```python
from build123d import *

# Parameters (mm, degrees)
SKETCH1_R           = 0.635
BOSS_EXTRUDE1_DEPTH = 1.27
FILLET1_R           = 0.254


with BuildPart() as part:
    # Sketch1 → Boss-Extrude1 (new body)
    with BuildSketch(Plane(origin=(0, 0, 0), x_dir=(1, 0, 0), z_dir=(0, 1, 0))):
        with BuildLine():
            ThreePointArc((-4.445, -13.249953655), (-4.662189736, -11.349360189), (-5.931882655, -9.9185189))
            ThreePointArc((-5.931882655, -9.9185189), (0, 11.557), (5.931882655, -9.9185189))
            ThreePointArc((5.931882655, -9.9185189), (4.662189736, -11.349360189), (4.445, -13.249953655))
            Line((4.445, -13.249953655), (1.27, -13.249953655))
            Line((1.27, -13.249953655), (1.27, -9.439953655))
            ThreePointArc((1.27, -9.439953655), (0, 9.525), (-1.27, -9.439953655))
            Line((-1.27, -9.439953655), (-1.27, -13.249953655))
            Line((-1.27, -13.249953655), (-4.445, -13.249953655))
        make_face()
        with Locations(Location((2.54, -11.725953655, 0), (0, 0, 270))):
            Circle(SKETCH1_R, mode=Mode.SUBTRACT)
        with Locations(Location((-2.54, -11.725953655, 0), (0, 0, 270))):
            Circle(SKETCH1_R, mode=Mode.SUBTRACT)
    extrude(amount=BOSS_EXTRUDE1_DEPTH)

    # Fillet1
    fillet1_edges = [part.edges().sort_by_distance(p)[0] for p in [
        (4.445, 0.635, 13.249953655),
        (-4.445, 0.635, 13.249953655),
    ]]
    fillet(fillet1_edges, radius=FILLET1_R)


solid = part.part
```
The listing builds one solid part. Answer for the finished solid, in the listing's coordinates (mm). A direction names the side the tool comes from. Coordinates: 2 decimals unless noted, no trailing zeros. Loops run counter-clockwise (first coordinate to the right, second up) from the corner with the lowest first, then second, coordinate; pieces in that order, holes last. Notation, with made-up numbers: M 42,0 L 83,0 A33 ccw 83,35 Z; hole C 76.25,-5.5 d7. An arc over 180 degrees is marked long. Answer as CSV lines item,"result". Start each with the question number.
(1) Find the intervals of material crossed by L1, parallel to Z at x = 3, y = 0.75; L2, parallel to X at y = 0.55, z = 0 (3 decimals); L3, parallel to X at y = 1.15, z = 10.5, in increasing order. Write a range as [from, to].
(2) The part is cut by section D-D (x = 2.54). Give the vertices of the cut face in (y, z), and give its area (3 significant figures).
(3) The mould has two halves that part along Z. Classify faces 1 (the flat face through (3, 1, 13.25)), 2 (the cylindrical face through (0.401, 0.626, -9.517)), 3 (the flat face through (9, 1.27, 4)), 4 (the cylindrical face through (-2.51, 0.63, 11.09)): pulls with the +Z half, pulls with the -Z half, needs draft (parallel to the pull), parting line crosses it, or undercut.
(4) The part is cut by section C-C (y = 0.5). Give the vertices of the cut face in (x, z) (3 decimals).
(5) For faces 5 (the cylindrical face through (-4.712, 0.626, 11.244)), 6 (the flat face through (-1.27, 1, 11)), determine the directions among +Z, -Z, +X, -X, +Y, -Y from which every point of the face is accessible in a straight line to the end or side of a thin tool.
(6) The part is cut by section B-B (x = -9.25). Give the vertices of the cut face in (y, z).
(7) The part is cut by section A-A (z = 0). Give the vertices of the cut face in (x, y) (3 decimals).
Determined:
1,L1,"[-11.16, -9.04], [9.04, 11.29], [12.16, 13.25]"
1,L2,"[-11.557, -9.525], [9.525, 11.557]"
1,L3,"[-5.22, -1.27], [1.27, 5.22]"
2,outline,"M 0,-11.27 L 1.27,-11.27 L 1.27,-9.18 L 0,-9.18 Z; M 0,9.18 L 1.27,9.18 L 1.27,11.09 L 0,11.09 Z; M 0,12.36 L 1.27,12.36 L 1.27,13.25 L 0,13.25 Z"
2,area,"6.22 mm2"
3,face 1,"pulls with the +Z half"
3,face 2,"undercut"
3,face 3,"needs draft"
3,face 4,"undercut"
4,outline,"M -5.932,9.919 A11.557 ccw long 5.932,9.919 A3.175 cw 4.403,12.97 A0.254 ccw 4.151,13.25 L 1.27,13.25 L 1.27,9.44 A9.525 cw long -1.27,9.44 L -1.27,13.25 L -4.151,13.25 A0.254 ccw -4.403,12.97 A3.175 cw Z; hole C -2.54,11.726 d1.27; hole C 2.54,11.726 d1.27"
5,face 5,"-X, +Y, -Y"
5,face 6,"+Z, +Y, -Y"
6,outline,"M 0,-6.93 L 1.27,-6.93 L 1.27,-2.27 L 0,-2.27 Z; M 0,2.27 L 1.27,2.27 L 1.27,6.93 L 0,6.93 Z"
7,outline,"M -11.557,0 L -9.525,0 L -9.525,1.27 L -11.557,1.27 Z; M 9.525,0 L 11.557,0 L 11.557,1.27 L 9.525,1.27 Z"
